Here's how the part is built. I have some questions about the finished solid (model axes, mm). Face numbers are marked on the shaded views. A direction names the side the tool comes from. Coordinates: 2 decimals unless noted, no trailing zeros. Write each loop counter-clockwise with the first axis right and the second up, starting at its lowest first coordinate (ties: lowest second). Pieces come first, ordered by that corner, then holes. Notation, with made-up numbers: (8.5, -28.75) - (55.5, -28.75) arc R22 ccw to (55.5, 10.25) - close; hole circle Ø7 at (-39, 58). An arc over 180 degrees is marked (long way). Answer in a Markdown table with one row per item. Add a question column.
Item 1: Imagine slicing it at C-C (y = 0). Please give me the cut outline in (x, z), plus the area to 3 significant figures.
Item 2: Imagine slicing it at A-A (x = -1). Please give me the cut outline in (y, z), plus the area to 3 significant figures.
Item 3: We'd pull the mould along Z, two halves only. Please class the marked faces 5, 6 and 7: +Z half, -Z half, draft (parallel to the pull), parting line (faces both ways), or undercut.
Item 4: Imagine slicing it at D-D (x = -14). Please give me the cut outline in (y, z).
Item 5: Which directions (+Z, -Z, +X, -X, +Y, -Y) give clear straight access to the entire face, cutting with the end or side of a thin tool? Please do the marked faces 1, 2, 3 and 4.
Item 6: Imagine slicing it at B-B (z = 6.25). Please give me the cut outline in (x, y), plus the area to 3 significant figures.
Item 7: If I drill on probe 1 along Y at (x, z) = (7.25, 4.75); probe 2 along Z at (x, y) = (7.75, -10); probe 3 along Y at (x, z) = (-3.5, 2.5), over which ranges is the centre line in solid material (lowest first)? Write a range as from..to.
Item 8: I'm going to push flat-ended pins straight in: pin 1 (5 mm diameter, centred on x = -14.5, z = 4.5, fed in from +Y); pin 2 (2.5 mm diameter, centred on x = -1, z = 5, fed in from -Y) (3 decimals); pin 3 (5 mm diameter, centred on x = -6.5, z = 7.5, fed in from -Y); pin 4 (2.5 mm diameter, centred on x = -15.5, y = -1.5, fed in from +Z). Where does each tip first touch, or does it pass through?
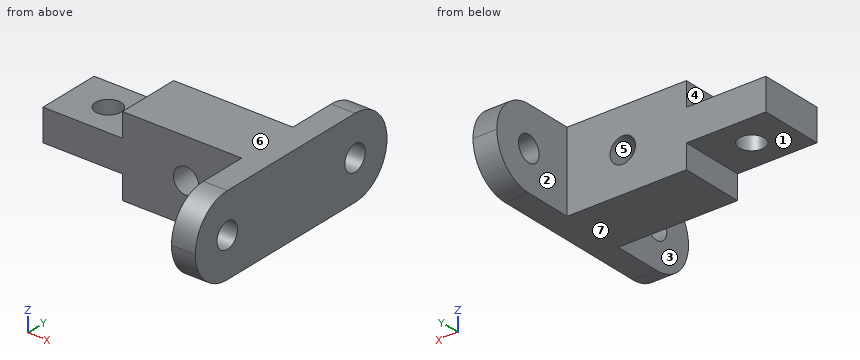
from build123d import *

# Parameters (mm, degrees)
BOSS_EXTRU_1_DEPTH      = 10
ESQUISSE2_R             = 1.6
ENL_V_MAT_EXTRU_1_DEPTH = 10
CONG_1_R                = 5
ESQUISSE3_W             = 10
ESQUISSE3_H             = 3
ENL_V_MAT_EXTRU_2_DEPTH = 10
ESQUISSE4_R             = 1.6
ENL_V_MAT_EXTRU_3_DEPTH = 10
ESQUISSE5_R             = 1.6
ENL_V_MAT_EXTRU_4_DEPTH = 10


with BuildPart() as part:
    # Esquisse1 → Boss.-Extru.1 (new body)
    with BuildSketch(Plane.XY):
        Polygon((6, -4), (6, -15), (9, -15), (9, 15), (6, 15), (6, 4), (-19, 4), (-19, -4), align=None)
    extrude(amount=BOSS_EXTRU_1_DEPTH)

    # Esquisse2 → Enlèv. mat.-Extru.1 (cut)
    with BuildSketch(Plane.ZY.offset(-6)):
        with Locations(Location((5, 10, 0), (0, 0, 270))):
            Circle(ESQUISSE2_R)
    enl_v_mat_extru_1 = extrude(amount=-ENL_V_MAT_EXTRU_1_DEPTH, mode=Mode.SUBTRACT)

    # Symétrie3: Enlèv. mat.-Extru.1 across plane
    add(enl_v_mat_extru_1.mirror(Plane.ZX), mode=Mode.SUBTRACT)

    # Congé1
    cong_1_edges = [part.edges().sort_by_distance(p)[0] for p in [
        (7.5, 15, 0),
        (7.5, 15, 10),
        (7.5, -15, 0),
        (7.5, -15, 10),
    ]]
    fillet(cong_1_edges, radius=CONG_1_R - 0.0001)  # a hair under: the kernel refuses the full size

    # Esquisse3 → Enlèv. mat.-Extru.2 (cut)
    with BuildSketch(Plane(origin=(0, 4, 0), x_dir=(1, 0, 0), z_dir=(0, 1, 0))):
        with Locations((-14, -1.5)):
            Rectangle(ESQUISSE3_W, ESQUISSE3_H)
        with Locations((-14, -8.5)):
            Rectangle(ESQUISSE3_W, ESQUISSE3_H)
    extrude(amount=-ENL_V_MAT_EXTRU_2_DEPTH, mode=Mode.SUBTRACT)

    # Esquisse4 → Enlèv. mat.-Extru.3 (cut)
    with BuildSketch(Plane(origin=(0, 0, 3), x_dir=(-1, 0, 0), z_dir=(0, 0, -1))):
        with Locations((14, 0)):
            Circle(ESQUISSE4_R)
    extrude(amount=-ENL_V_MAT_EXTRU_3_DEPTH, mode=Mode.SUBTRACT)

    # Esquisse5 → Enlèv. mat.-Extru.4 (cut)
    with BuildSketch(Plane.XZ.offset(4)):
        with Locations((-1, 5)):
            Circle(ESQUISSE5_R)
    extrude(amount=-ENL_V_MAT_EXTRU_4_DEPTH, mode=Mode.SUBTRACT)


solid = part.part
Here are the results:
| question | item | result |
|---|---|---|
| 1 | outline | (-19, 3) - (-15.6, 3) - (-15.6, 7) - (-19, 7) - close; (-12.4, 3) - (-9, 3) - (-9, 0) - (9, 0) - (9, 10) - (-9, 10) - (-9, 7) - (-12.4, 7) - close; hole circle Ø3.2 at (-1, 5) |
| 1 | area | 199 mm2 |
| 2 | outline | (-4, 0) - (4, 0) - (4, 3.4) - (-4, 3.4) - close; (-4, 6.6) - (4, 6.6) - (4, 10) - (-4, 10) - close |
| 2 | area | 54.4 mm2 |
| 3 | face 5 | undercut |
| 3 | face 6 | +Z half |
| 3 | face 7 | -Z half |
| 4 | outline | (-4, 3) - (-1.6, 3) - (-1.6, 7) - (-4, 7) - close; (1.6, 3) - (4, 3) - (4, 7) - (1.6, 7) - close |
| 5 | face 1 | -Z, -X, +Y, -Y |
| 5 | face 2 | +Z, -Z, -X, +Y |
| 5 | face 3 | +Z, -Z, -X, -Y |
| 5 | face 4 | +Z, -X, +Y, -Y |
| 6 | outline | (-19, -4) - (-2, -4) - (-2, 4) - (-19, 4) - close; (0, -4) - (6, -4) - (6, -9) - (9, -9) - (9, 9) - (6, 9) - (6, 4) - (0, 4) - close; (6, -14.84) - (9, -14.84) - (9, -11) - (6, -11) - close; (6, 11) - (9, 11) - (9, 14.84) - (6, 14.84) - close; hole circle Ø3.2 at (-14, 0) |
| 6 | area | 253 mm2 |
| 7 | probe 1 | y = -14.99..-11.58, -8.42..8.42, 11.58..14.99 |
| 7 | probe 2 | z = 0..3.4, 6.6..10 |
| 7 | probe 3 | y = -4..4 |
| 8 | pin 1 | stops at y = 4 |
| 8 | pin 2 | passes through |
| 8 | pin 3 | stops at y = -4 |
| 8 | pin 4 | stops at z = 7 |
